The listing builds one solid part. Answer for the finished solid, in the listing's coordinates (mm). Face numbers are marked on the shaded views. A direction names the side the tool comes from. Round coordinates to 2 decimals unless told otherwise and drop trailing zeros. One line per item, written item: value.
```python
from build123d import *

# Parameters (mm, degrees)
SKETCH2_W                                 = 159
SKETCH2_H                                 = 95
BASE_EXTRUDE_DEPTH                        = 16
BOSS_EXTRUDE1_DEPTH                       = 16
BOSS_EXTRUDE2_REACH                       = 122.054
SKETCH4_R                                 = 31.5
RIB1_REACH                                = 126.027
SKETCH5_WALL_W                            = 278.31185129
SKETCH5_WALL_H                            = 13
BOSS_EXTRUDE3_DEPTH                       = 16
SKETCH7_R                                 = 6.25
CUT_EXTRUDE1_DEPTH                        = 139.006210257
FILLET1_R                                 = 12.5
CUT_EXTRUDE2_START                        = -5
CUT_EXTRUDE2_DEPTH                        = 5
RIB2_REACH                                = 153.878
SKETCH9_WALL_W                            = 345.396032214
SKETCH9_WALL_H                            = 5
CBORE_FOR_M24_HEX_HEAD_SCREW1_D           = 26
CBORE_FOR_M24_HEX_HEAD_SCREW1_CBORE_D     = 44.569
CBORE_FOR_M24_HEX_HEAD_SCREW1_CBORE_DEPTH = 15
FILLET4_R                                 = 6
CUT_EXTRUDE3_REACH                        = 143.476
SKETCH13_R                                = 6.25


with BuildPart() as part:
    # Sketch2 → Base-Extrude (new body)
    with BuildSketch(Plane(origin=(0, 0, 0), x_dir=(1, 0, 0), z_dir=(0, 1, 0))):
        Rectangle(SKETCH2_W, SKETCH2_H)
    extrude(amount=BASE_EXTRUDE_DEPTH)

    # Sketch3 → Boss-Extrude1 (add)
    with BuildSketch(Plane(origin=(-26.80320323, 46.4245098, 0), x_dir=(0, 0, -1), z_dir=(0.499999999999998, -0.8660254037844398, 0))):
        with BuildLine():
            Line((-19, -60.849019601), (-19, 1.242015055))
            ThreePointArc((-19, 1.242015055), (0, 72.150980399), (19, 1.242015055))
            Line((19, 1.242015055), (19, -60.849019601))
            Line((19, -60.849019601), (-19, -60.849019601))
        make_face()
    extrude(amount=BOSS_EXTRUDE1_DEPTH)

    # Boss-Extrude2: up to this plane
    boss_extrude2_end = Plane(origin=(-79.5, 16, -47.5), z_dir=(0, -1, 0))
    # Sketch4 → Boss-Extrude2 (add, up to the surface)
    with BuildSketch(Plane(origin=(-18.80320323, 32.56810334, 0), x_dir=(0.8660254037844398, 0.49999999999999806, 0), z_dir=(0.499999999999998, -0.8660254037844397, 0)), mode=Mode.PRIVATE) as boss_extrude2_sk1:
        with Locations(Location((34.150980399, 0, 0), (0, 0, 180))):
            Circle(SKETCH4_R)
    boss_extrude2_tool1 = split(extrude(boss_extrude2_sk1.sketch, amount=BOSS_EXTRUDE2_REACH, mode=Mode.PRIVATE), bisect_by=boss_extrude2_end, keep=Keep.BOTH, mode=Mode.PRIVATE)
    add(boss_extrude2_tool1.solids().sort_by_distance((10.772413, 49.643594, 0))[0])

    # Sketch5 wall → Rib1 (add, up to next)
    with BuildSketch(Plane(origin=(-22.439717295, 16, 0), x_dir=(1, 0, 0), z_dir=(0, 1, 0)), mode=Mode.PRIVATE) as rib1_sk1:
        Rectangle(SKETCH5_WALL_W, SKETCH5_WALL_H)
    rib1_tool1 = extrude(rib1_sk1.sketch, amount=RIB1_REACH, mode=Mode.PRIVATE) - part.part
    add(rib1_tool1.solids().sort_by_distance((-22.439717295, 16, 0))[0])

    # Sketch6 → Boss-Extrude3 (add)
    with BuildSketch(Plane(origin=(-26.80320323, 46.4245098, 0), x_dir=(-0.8660254037844398, -0.49999999999999806, 0), z_dir=(-0.499999999999998, 0.8660254037844397, 0))):
        with BuildLine():
            Line((-18.150980399, 34.467375879), (-18.150980399, 67))
            ThreePointArc((-18.150980399, 67), (-34.150980399, 83), (-50.150980399, 67))
            Line((-50.150980399, 67), (-50.150980399, 34.467375879))
            ThreePointArc((-50.150980399, 34.467375879), (-34.150980399, 38), (-18.150980399, 34.467375879))
        make_face()
    extrude(amount=-BOSS_EXTRUDE3_DEPTH)

    # Sketch7 → Cut-Extrude1 (cut, through all)
    with BuildSketch(Plane(origin=(-18.80320323, 32.56810334, 0), x_dir=(-0.8660254037844398, -0.49999999999999806, 0), z_dir=(-0.499999999999998, 0.8660254037844397, 0))):
        with Locations(Location((-34.150980399, 67, 0), (0, 0, 180))):
            Circle(SKETCH7_R)
    extrude(amount=CUT_EXTRUDE1_DEPTH, mode=Mode.SUBTRACT)

    # Fillet1
    fillet1_edges = [part.edges().sort_by_distance(p)[0] for p in [
        (-21.72758664, 40.117314098, 19),
        (-21.72758664, 40.117314098, -19),
        (20.62881982, 64.57179677, 34.467375879),
        (-7.083993101, 48.57179677, 34.467375879),
        (-79.5, 8, -47.5),
        (79.5, 8, -47.5),
        (79.5, 8, 47.5),
        (-79.5, 8, 47.5),
    ]]
    fillet(fillet1_edges, radius=FILLET1_R)

    # Sketch8 → Cut-Extrude2 (cut)
    with BuildSketch(Plane.XZ.offset(CUT_EXTRUDE2_START)):
        with BuildLine():
            Line((-51.793093674, -35), (51.793093674, -35))
            ThreePointArc((51.793093674, -35), (53.698095579, -34.317534842), (54.736365866, -32.580645161))
            ThreePointArc((54.736365866, -32.580645161), (58.161165235, -26.161165235), (64.580645161, -22.736365866))
            ThreePointArc((64.580645161, -22.736365866), (66.317534842, -21.698095579), (67, -19.793093674))
            Line((67, -19.793093674), (67, 19.793093674))
            ThreePointArc((67, 19.793093674), (66.317534842, 21.698095579), (64.580645161, 22.736365866))
            ThreePointArc((64.580645161, 22.736365866), (58.161165235, 26.161165235), (54.736365866, 32.580645161))
            ThreePointArc((54.736365866, 32.580645161), (53.698095579, 34.317534842), (51.793093674, 35))
            Line((51.793093674, 35), (-51.793093674, 35))
            ThreePointArc((-51.793093674, 35), (-53.698095579, 34.317534842), (-54.736365866, 32.580645161))
            ThreePointArc((-54.736365866, 32.580645161), (-58.161165235, 26.161165235), (-64.580645161, 22.736365866))
            ThreePointArc((-64.580645161, 22.736365866), (-66.317534842, 21.698095579), (-67, 19.793093674))
            Line((-67, 19.793093674), (-67, -19.793093674))
            ThreePointArc((-67, -19.793093674), (-66.317534842, -21.698095579), (-64.580645161, -22.736365866))
            ThreePointArc((-64.580645161, -22.736365866), (-58.161165235, -26.161165235), (-54.736365866, -32.580645161))
            ThreePointArc((-54.736365866, -32.580645161), (-53.698095579, -34.317534842), (-51.793093674, -35))
        make_face()
    extrude(amount=CUT_EXTRUDE2_DEPTH, mode=Mode.SUBTRACT)

    # Sketch9 wall → Rib2 (add, up to next)
    with BuildSketch(Plane(origin=(18.77241336, 35.787187078, 42.302042556), x_dir=(-0.40362765533, 0.699103606369, 0.590202391909), z_dir=(-0.295101195954, 0.511130264767, -0.807255310658)), mode=Mode.PRIVATE) as rib2_sk1:
        Rectangle(SKETCH9_WALL_W, SKETCH9_WALL_H)
    rib2_tool1 = extrude(rib2_sk1.sketch, amount=RIB2_REACH, mode=Mode.PRIVATE) - part.part
    add(rib2_tool1.solids().sort_by_distance((18.77241336, 35.787187078, 42.302042556))[0])

    # CBORE for M24 Hex Head Screw1 (through all)
    with Locations(Plane(origin=(-26.80320323, 46.4245098, 0), x_dir=(-0.8660254037844398, -0.49999999999999806, 0), z_dir=(-0.499999999999998, 0.8660254037844397, 0))):
        with Locations((-34.150980399, 0)):
            CounterBoreHole(CBORE_FOR_M24_HEX_HEAD_SCREW1_D / 2, CBORE_FOR_M24_HEX_HEAD_SCREW1_CBORE_D / 2, CBORE_FOR_M24_HEX_HEAD_SCREW1_CBORE_DEPTH)

    # Fillet4
    fillet4_edges = [part.edges().sort_by_distance(p)[0] for p in [
        (-47.5, 16, -12.75),
        (-47.5, 16, 12.75),
    ]]
    fillet(fillet4_edges, radius=FILLET4_R)

    # Sketch13 → Cut-Extrude3 (cut, up to next)
    with BuildSketch(Plane.XZ, mode=Mode.PRIVATE) as cut_extrude3_sk1:
        with Locations(Location((67, 35, 0), (0, 0, 270))):
            Circle(SKETCH13_R)
    cut_extrude3_tool1 = extrude(cut_extrude3_sk1.sketch, amount=-CUT_EXTRUDE3_REACH, mode=Mode.PRIVATE) & part.part
    # Sketch13 → Cut-Extrude3 (cut, up to next)
    with BuildSketch(Plane.XZ, mode=Mode.PRIVATE) as cut_extrude3_sk2:
        with Locations(Location((67, -35, 0), (0, 0, 270))):
            Circle(SKETCH13_R)
    cut_extrude3_tool2 = extrude(cut_extrude3_sk2.sketch, amount=-CUT_EXTRUDE3_REACH, mode=Mode.PRIVATE) & part.part
    # Sketch13 → Cut-Extrude3 (cut, up to next)
    with BuildSketch(Plane.XZ, mode=Mode.PRIVATE) as cut_extrude3_sk3:
        with Locations(Location((-67, -35, 0), (0, 0, 270))):
            Circle(SKETCH13_R)
    cut_extrude3_tool3 = extrude(cut_extrude3_sk3.sketch, amount=-CUT_EXTRUDE3_REACH, mode=Mode.PRIVATE) & part.part
    # Sketch13 → Cut-Extrude3 (cut, up to next)
    with BuildSketch(Plane.XZ, mode=Mode.PRIVATE) as cut_extrude3_sk4:
        with Locations(Location((-67, 35, 0), (0, 0, 270))):
            Circle(SKETCH13_R)
    cut_extrude3_tool4 = extrude(cut_extrude3_sk4.sketch, amount=-CUT_EXTRUDE3_REACH, mode=Mode.PRIVATE) & part.part
    add(cut_extrude3_tool1.solids().sort_by_distance((67, 0, 35))[0], mode=Mode.SUBTRACT)
    add(cut_extrude3_tool2.solids().sort_by_distance((67, 0, -35))[0], mode=Mode.SUBTRACT)
    add(cut_extrude3_tool3.solids().sort_by_distance((-67, 0, -35))[0], mode=Mode.SUBTRACT)
    add(cut_extrude3_tool4.solids().sort_by_distance((-67, 0, 35))[0], mode=Mode.SUBTRACT)


solid = part.part
```
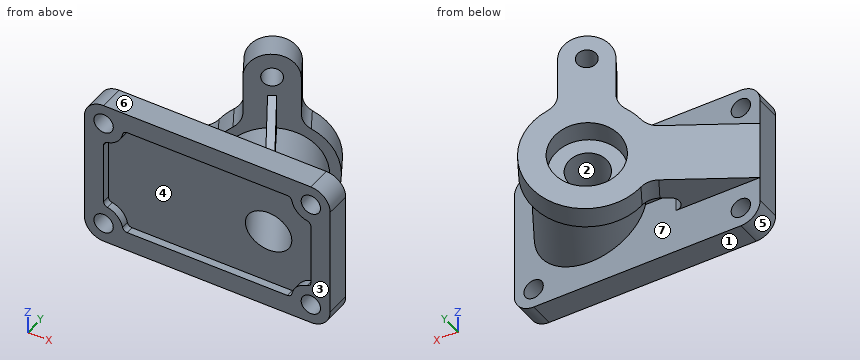
1) For the marked faces 5, 6 and 7, determine the directions among +Z, -Z, +X, -X, +Y, -Y from which every point of the face is accessible in a straight line to the end or side of a thin tool.
Final values:
face 5: -Z, -X, +Y, -Y
face 6: +Z, +X, -X, -Y
face 7: none
2) Consider L1, parallel to X at y = 9.25, z = -35; L2, parallel to Y at x = -31, z = -40; L3, parallel to Y at x = 43, z = -5. Determine where each line is inside the solid, lowest interval first.
Final values:
L1: -79.5 to -73.25, -60.75 to 60.75, 73.25 to 79.5
L2: 0 to 16
L3: 17.82 to 56.03, 68.25 to 69.16
3) For a pull along Z with two mould halves and no side action, classify the marked faces 1, 2, 3 and 4 as released by +Z, released by -Z, zero draft, split by the parting line, or undercut.
Final values:
face 1: released by -Z
face 2: undercut
face 3: zero draft
face 4: undercut
4) Each of these flat-tipped pins is pushed along its axis until it touches: pin 1 Ø3 at (x, y) = (-25.5, 20) entering from -Z; pin 2 Ø2 at (x, z) = (47.5, -1) entering from -Y; pin 3 Ø5 at (x, y) = (18, 8.5) entering from +Z; pin 4 Ø11 at (x, z) = (67, 35) entering from -Y. Where does it stop, or does it pass through?
Final values:
pin 1: z = -6.5
pin 2: y = 10.21
pin 3: z = 47.5
pin 4: through
